Read the model definition and answer for the solid it produces. Units are mm, in the model's axes. Face numbers are marked on the shaded views. A direction names the side the tool comes from. Round coordinates to 2 decimals unless told otherwise and drop trailing zeros. Order: outer loops, then holes, each group sorted by start corner. A loop starts at its lowest first (then second) coordinate and runs counter-clockwise, first axis right, second up. Notation, with made-up numbers: (71, 61.25) -> (79, 61.25) arc R21 cw to (79, 97.25) -> close; hole circle Ø7 at (-21.5, -7). An arc over 180 degrees is marked (long way). Use a Markdown table: item, result. Add a question column.
1. Consider L1, parallel to Y at x = 0, z = 8.5; L2, parallel to Y at x = 0, z = 3.85; L3, parallel to Y at x = -1, z = 11. Determine where each line is inside the solid, lowest interval first. Write a range as [from, to].
2. Given pin 1 (3 mm diameter, centred on x = 3, y = 12, fed in from +Z); pin 2 (6 mm diameter, centred on x = -1, z = 10.5, fed in from -Y); pin 3 (5 mm diameter, centred on x = 0, y = -11.23, fed in from -Z), each flat-ended and moving along its own axis, determine where each tip first touches the part or whether it passes through.
3. For the marked faces 1, 2 and 3, determine the directions among +Z, -Z, +X, -X, +Y, -Y from which every point of the face is accessible in a straight line to the end or side of a thin tool.
4. Section C-C, the plane z = 2.25 is taken. Give the vertices of the cut face in (x, y) (3 decimals), then the cut area to 3 significant figures.
5. Section A-A, the plane z = 7.25 is taken. Give the number of separate pieces and of enclosed holes in the cut face, then the cut area to 3 significant figures.
6. The mould has two halves that part along Y. Classify the marked faces 4, 5 and 6: +Y half, -Y half, draft (parallel to the pull), parting line (faces both ways), or undercut.
7. Section D-D, the plane y = -4 is taken. Give the vertices of the cut face in (x, z) (3 decimals).
8. Section B-B, the plane x = 0 is taken. Give the vertices of the cut face in (y, z), then the cut area to 3 significant figures.
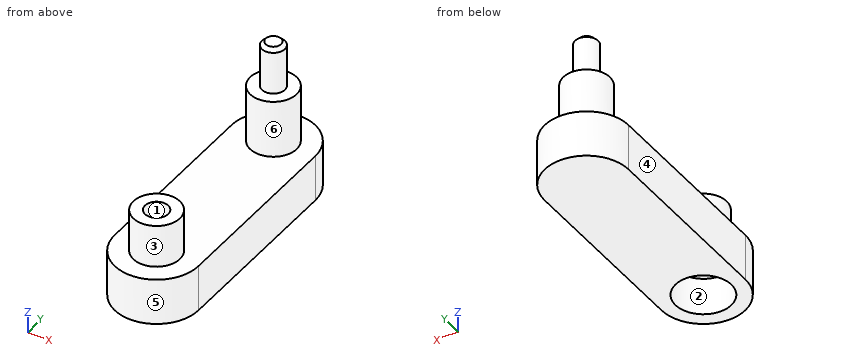
```python
from build123d import *

# Parameters (mm, degrees)
F1_DEPTH  = 6.35
F2_R      = 3.175
F3_DEPTH  = 7.874
F4_R      = 1.5621
F5_DEPTH  = 6.35
F6_SIZE   = 0.508
F7_R      = 3.175
F8_DEPTH  = 5.842
F9_R      = 1.5875
F10_DEPTH = 12.193
F11_R     = 3.81
F12_DEPTH = 5.08


with BuildPart() as f1:
    # F0 (on Top) → F1 (new body)
    with BuildSketch(Plane.XY):
        with BuildLine():
            ThreePointArc((5.715, 14.162212), (0, 19.877212), (-5.715, 14.162212))
            Line((-5.715, 14.162212), (-5.715, -11.231923))
            ThreePointArc((-5.715, -11.231923), (0, -16.946923), (5.715, -11.231923))
            Line((5.715, -11.231923), (5.715, 14.162212))
        make_face()
    extrude(amount=F1_DEPTH)

    # F2 (on face) → F3 (join)
    with BuildSketch(Plane.XY.offset(6.35)):
        with Locations((0, 14.162212)):
            Circle(F2_R)
    extrude(amount=F3_DEPTH)

    # F4 (on face) → F5 (join)
    with BuildSketch(Plane.XY.offset(14.224)):
        with Locations((0, 14.162212)):
            Circle(F4_R)
    extrude(amount=F5_DEPTH)

    # F6
    f6_edges = [f1.edges().sort_by_distance(p)[0] for p in [
        (-1.5621, 14.162212, 20.574),
    ]]
    chamfer(f6_edges, length=F6_SIZE)

    # F7 (on face) → F8 (join)
    with BuildSketch(Plane.XY.offset(6.35)):
        with Locations((0, -11.231923)):
            Circle(F7_R)
    extrude(amount=F8_DEPTH)

    # F9 (on face) → F10 (cut, through all)
    with BuildSketch(Plane.XY.offset(12.192)):
        with Locations((0, -11.231923)):
            Circle(F9_R)
    extrude(amount=-F10_DEPTH, mode=Mode.SUBTRACT)

    # F11 (on face) → F12 (cut)
    with BuildSketch(Plane(origin=(0, 0, 0), x_dir=(1, 0, 0), z_dir=(0, 0, -1))):
        with Locations((0, 11.231923)):
            Circle(F11_R)
    extrude(amount=-F12_DEPTH, mode=Mode.SUBTRACT)


solid = f1.part
```
Verdict:
| question | item | result |
|---|---|---|
| 1 | L1 | y = [-14.41, -12.82], [-9.64, -8.06], [10.99, 17.34] |
| 1 | L2 | y = [-16.95, -15.04], [-7.42, 19.88] |
| 1 | L3 | y = [-14.25, -12.46], [-10, -8.22], [11.15, 17.18] |
| 2 | pin 1 | stops at z = 14.22 |
| 2 | pin 2 | stops at y = -14.41 |
| 2 | pin 3 | stops at z = 5.08 |
| 3 | face 1 | +Z, -Z |
| 3 | face 2 | -Z |
| 3 | face 3 | +Z |
| 4 | outline | (-5.715, -11.232) arc R5.715 ccw to (5.715, -11.232) -> (5.715, 14.162) arc R5.715 ccw to (-5.715, 14.162) -> close; hole circle Ø7.62 at (0, -11.232) |
| 4 | area | 347 mm2 |
| 5 | separate pieces | 2 |
| 5 | enclosed holes | 1 |
| 5 | area | 55.4 mm2 |
| 6 | face 4 | draft |
| 6 | face 5 | -Y half |
| 6 | face 6 | undercut |
| 7 | outline | (-5.715, 0) -> (5.715, 0) -> (5.715, 6.35) -> (-5.715, 6.35) -> close |
| 8 | outline | (-16.95, 0) -> (-15.04, 0) -> (-15.04, 5.08) -> (-12.82, 5.08) -> (-12.82, 12.19) -> (-14.41, 12.19) -> (-14.41, 6.35) -> (-16.95, 6.35) -> close; (-9.64, 5.08) -> (-7.42, 5.08) -> (-7.42, 0) -> (19.88, 0) -> (19.88, 6.35) -> (17.34, 6.35) -> (17.34, 14.22) -> (15.72, 14.22) -> (15.72, 20.07) -> (15.22, 20.57) -> (13.11, 20.57) -> (12.6, 20.07) -> (12.6, 14.22) -> (10.99, 14.22) -> (10.99, 6.35) -> (-8.06, 6.35) -> (-8.06, 12.19) -> (-9.64, 12.19) -> close |
| 8 | area | 279 mm2 |
